```python
from build123d import *

# Parameters (mm, degrees)
SALIENTE_EXTRUIR5_DEPTH = 12.5
CROQUIS10_W             = 18
CROQUIS10_H             = 53
CORTAR_EXTRUIR1_DEPTH   = 8.5
CROQUIS11_R             = 4
CORTAR_EXTRUIR2_DEPTH   = 8
CROQUIS12_2_R           = 3
CORTAR_EXTRUIR3_DEPTH   = 8.7


with BuildPart() as part:
    # Croquis1 → Saliente-Extruir5 (new body)
    with BuildSketch(Plane.XY):
        with BuildLine():
            Line((-19.284730396, -35), (19.284730396, -35))
            add(Edge.make_bspline(
                [(19.284730396, -35), (25, -19.758503488), (25, 0)],
                knots=[0.881021326, 0.881021326, 0.881021326, 1.570796327, 1.570796327, 1.570796327], degree=2, weights=[1, 0.941113494, 1]))
            ThreePointArc((25, 0), (0, 25), (-25, 0))
            add(Edge.make_bspline(
                [(-25, 0), (-25, -19.758503488), (-19.284730396, -35)],
                knots=[4.71238898, 4.71238898, 4.71238898, 5.402163981, 5.402163981, 5.402163981], degree=2, weights=[1, 0.941113494, 1]))
        make_face()
    extrude(amount=SALIENTE_EXTRUIR5_DEPTH)

    # Croquis10 → Cortar-Extruir1 (cut)
    with BuildSketch(Plane.XY.offset(12.5)):
        with Locations((0, -5.5)):
            Rectangle(CROQUIS10_W, CROQUIS10_H)
    extrude(amount=-CORTAR_EXTRUIR1_DEPTH, mode=Mode.SUBTRACT)

    # Croquis11 → Cortar-Extruir2 (cut)
    with BuildSketch(Plane.XZ.offset(35)):
        with Locations((0, 12.5)):
            Circle(CROQUIS11_R)
    extrude(amount=-CORTAR_EXTRUIR2_DEPTH, mode=Mode.SUBTRACT)

    # Croquis12<2> → Cortar-Extruir3 (cut)
    with BuildSketch(Plane.XY.offset(12.5)):
        with Locations((16, -20)):
            Circle(CROQUIS12_2_R)
        with Locations((16, 10)):
            Circle(CROQUIS12_2_R)
        with Locations((-18, -5)):
            Circle(CROQUIS12_2_R)
        with Locations((18, -5)):
            Circle(CROQUIS12_2_R)
        with Locations((-16, -20)):
            Circle(CROQUIS12_2_R)
        with Locations((-16, 10)):
            Circle(CROQUIS12_2_R)
    extrude(amount=-CORTAR_EXTRUIR3_DEPTH, mode=Mode.SUBTRACT)


solid = part.part
```
For this review, take the finished solid that the model builds, in its own axes (mm). A direction names the side the tool comes from. Round coordinates to 2 decimals unless told otherwise and drop trailing zeros. Loops run counter-clockwise (first coordinate to the right, second up) from the corner with the lowest first, then second, coordinate; pieces in that order, holes last.
Q1. Add section B-B on y = 15. Write out the cut boundary in (x, z).
Result sheet:
outline: (-20, 0) - (20, 0) - (20, 12.5) - (9, 12.5) - (9, 4) - (-9, 4) - (-9, 12.5) - (-20, 12.5) - close
Q2. Machinability: for faces 4 (the face through (-0.1, -33.5, 8.5)), 5 (the face through (0, -5, 0)), 6 (the face through (18, -5, 3.8)), which of the approach directions +Z, -Z, +X, -X, +Y, -Y give a long, thin tool a straight path to every point of the face, cutting with its end or side? Answer none if there is none.
Result sheet:
face 4: +Z, -Y
face 5: -Z, +X, -X, +Y, -Y
face 6: +Z
Q3. Add section D-D on x = -17. Write out the cut boundary in (y, z), plus the area to 3 significant figures.
Result sheet:
outline: (-35, 0) - (18.33, 0) - (18.33, 12.5) - (12.83, 12.5) - (12.83, 3.8) - (7.17, 3.8) - (7.17, 12.5) - (-2.17, 12.5) - (-2.17, 3.8) - (-7.83, 3.8) - (-7.83, 12.5) - (-17.17, 12.5) - (-17.17, 3.8) - (-22.83, 3.8) - (-22.83, 12.5) - (-35, 12.5) - close
area: 519 mm2
Q4. Mouldability with a two-part tool opening along Y and no side actions: class faces 1 (the face through (0, -35, 6)), 2 (the face through (13.6, 8.2, 8.2)), 3 (the face through (11, -5, 12.5)) as +Y half, -Y half, draft (parallel to the pull), parting line (faces both ways), or undercut.
Result sheet:
face 1: -Y half
face 2: undercut
face 3: draft
Q5. Add section A-A on x = 0. Write out the cut boundary in (y, z), plus the area to 4 significant figures.
Result sheet:
outline: (-35, 0) - (25, 0) - (25, 12.5) - (21, 12.5) - (21, 4) - (-32, 4) - (-32, 8.5) - (-35, 8.5) - close
area: 287.5 mm2
Q6. Add section C-C on z = 6.5. Give the number of separate pieces and of enclosed holes in the cut face, plus the area to 3 significant figures.
Result sheet:
separate pieces: 1
enclosed holes: 7
area: 1,480 mm2
Q7. Insertion check: pin 1 Ø3 at (x, y) = (-18, -5) entering from +Z; pin 2 Ø9 at (x, y) = (-2.5, -15.5) entering from +Z; pin 3 Ø3 at (y, z) = (-17.5, 7.5) entering from +X. Each pin has a flat end and moves straight along its axis. Give the tip position at first contact, or say it passes through.
Result sheet:
pin 1: stops at z = 3.8
pin 2: stops at z = 4
pin 3: stops at x = 23.92
Q8. To check wall thickness, follow line 1 along X through (y, z) = (-22.5, 6.5); line 2 along Y through (x, z) = (-16, 7.5); line 3 along X through (y, z) = (-18, 6.25). State the ranges of each line that lie inside material, in increasing order.
Result sheet:
line 1: x = -22.81 to -17.66, -14.34 to -9, 9 to 14.34, 17.66 to 22.81
line 2: y = -35 to -23, -17 to -7.24, -2.76 to 7, 13 to 19.21
line 3: x = -23.62 to -18.24, -13.76 to -9, 9 to 13.76, 18.24 to 23.62
